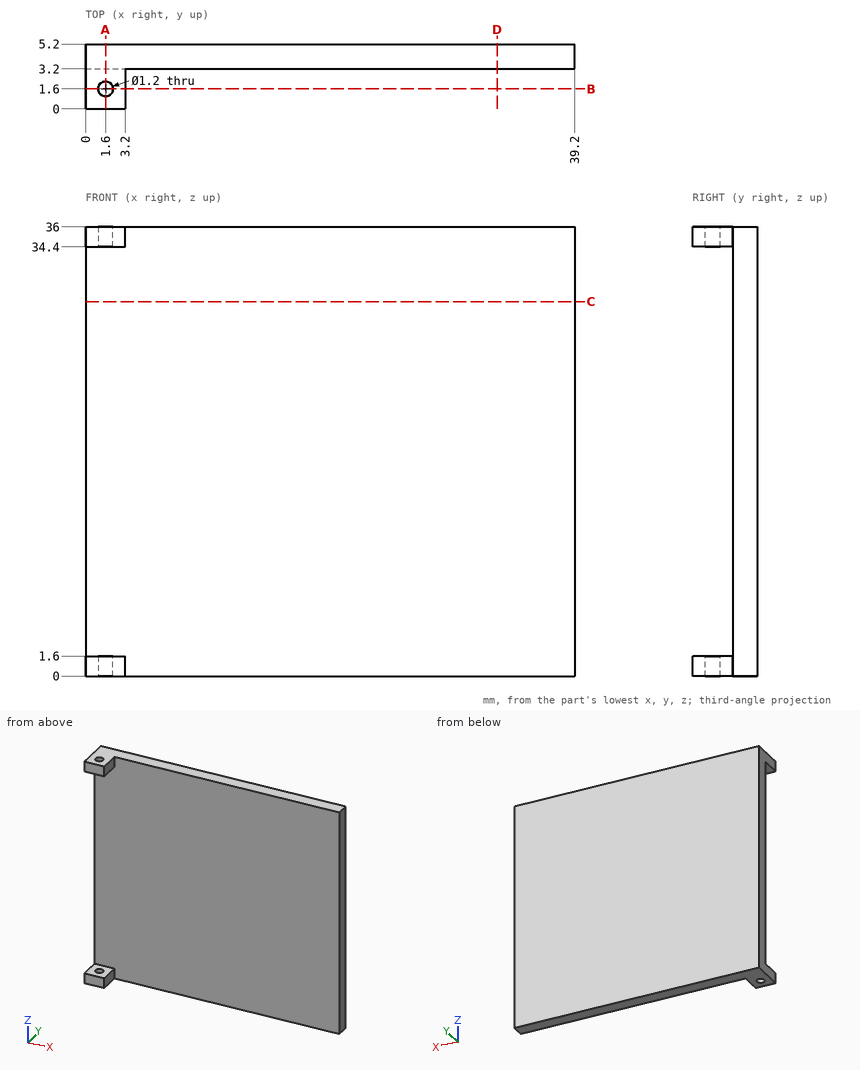
Job drawing, mm, ordinate dimensions from the low corner. One solid piece. Coordinates: 2 decimals unless noted, no trailing zeros. Loops run counter-clockwise (first coordinate to the right, second up) from the corner with the lowest first, then second, coordinate; pieces in that order, holes last. Notation, with made-up numbers: (-37, -10.5) -> (8, -10.5) arc R15 cw to (8, 13.5) -> close; hole circle Ø11 at (22, 14). An arc over 180 degrees is marked (long way). One line per item, written item: value.
1. Slice it at C-C on z = 30. Write the cut outline in (x, y).
Answers:
outline: (0, 3.2) -> (39.2, 3.2) -> (39.2, 5.2) -> (0, 5.2) -> close
2. Flat gauge pins, fed straight in: P1, Ø0.8, axis at y = 2.5, z = 35.5, coming from the +X side; P2, Ø11, axis at x = 19.5, z = 18.5, coming from the -Y side. Where does each tip first touch, or does it go through?
Answers:
P1: stops at x = 3.2
P2: stops at y = 3.2
3. Slice it at D-D on x = 33. Write the cut outline in (y, z).
Answers:
outline: (3.2, 0) -> (5.2, 0) -> (5.2, 36) -> (3.2, 36) -> close
4. Slice it at B-B on y = 1.6. Write the cut outline in (x, z), and give its area (3 significant figures).
Answers:
outline: (0, 0) -> (1, 0) -> (1, 1.6) -> (0, 1.6) -> close; (0, 34.4) -> (1, 34.4) -> (1, 36) -> (0, 36) -> close; (2.2, 0) -> (3.2, 0) -> (3.2, 1.6) -> (2.2, 1.6) -> close; (2.2, 34.4) -> (3.2, 34.4) -> (3.2, 36) -> (2.2, 36) -> close
area: 6.40 mm^2
5. Slice it at A-A on x = 1.6. Write the cut outline in (y, z), and give its area (3 significant figures).
Answers:
outline: (0, 0) -> (1, 0) -> (1, 1.6) -> (0, 1.6) -> close; (0, 34.4) -> (1, 34.4) -> (1, 36) -> (0, 36) -> close; (2.2, 0) -> (5.2, 0) -> (5.2, 36) -> (2.2, 36) -> (2.2, 34.4) -> (3.2, 34.4) -> (3.2, 1.6) -> (2.2, 1.6) -> close
area: 78.4 mm^2
6. Drill centre lines: line 1 (X direction, y = 1.6, z = 35.55); line 2 (Y direction, x = 1.6, z = 35.15); line 3 (Y direction, x = 5.5, z = 7.5). Where is each one in solid material? Low to high. Write a range as [from, to].
Answers:
line 1: x = [0, 1], [2.2, 3.2]
line 2: y = [0, 1], [2.2, 5.2]
line 3: y = [3.2, 5.2]
